Build history of the part. All positions in model axes, mm. Face numbers are marked on the shaded views. A direction names the side the tool comes from. Coordinates: 2 decimals unless noted, no trailing zeros. Loops run counter-clockwise (first coordinate to the right, second up) from the corner with the lowest first, then second, coordinate; pieces in that order, holes last. Notation, with made-up numbers: (39.5, -39) - (85.5, -39) arc R20 cw to (85.5, -4) - close; hole circle Ø3 at (-36, 86.25). An arc over 180 degrees is marked (long way). One line per item, written item: value.
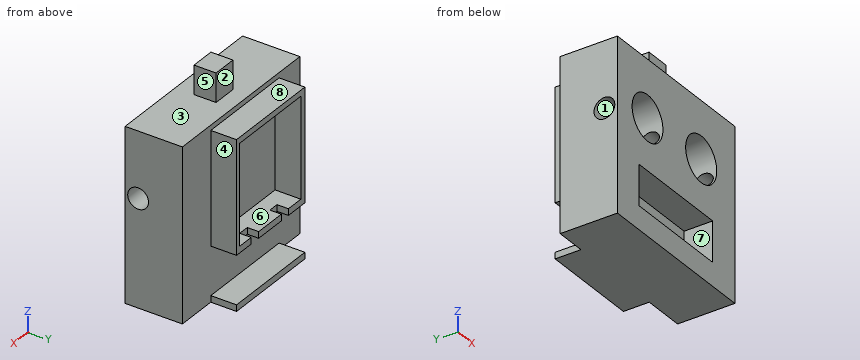
```python
from build123d import *

# Parameters (mm, degrees)
F0_W      = 76.2
F0_H      = 76.2
F1_DEPTH  = 25.4
F2_R      = 9.9906314399
F2_R_2    = 10.0773114698
F3_DEPTH  = 12.7
F4_W      = 47.7757537737
F4_H      = 17.8439570591
F5_DEPTH  = 12.7
F6_R      = 4.6109216101
F7_DEPTH  = 127
F8_W      = 44.3220883608
F8_H      = 49.7903954238
F9_DEPTH  = 11.43
F10_W     = 39.717190899
F10_H     = 44.3220883608
F11_DEPTH = 11.43
F12_W     = 44.3220883608
F12_H     = 2.8436683783
F13_DEPTH = 11.43
F14_W     = 4.6048909426
F14_H     = 2.8780568391
F14_W_2   = 4.8926984891
F15_DEPTH = 5.08
F16_W     = 10.9366197139
F16_H     = 9.7684562206
F17_DEPTH = 12.7


with BuildPart() as f1:
    # F0 (on Front) → F1 (new body)
    with BuildSketch(Plane.XZ):
        with Locations((-10.2171050385, 1.5830600848)):
            Rectangle(F0_W, F0_H)
    extrude(amount=-F1_DEPTH)

    # F2 (on face) → F3 (cut)
    with BuildSketch(Plane.XZ):
        with Locations((-28.7805758417, 14.3902888522)):
            Circle(F2_R)
        with Locations((6.0439212248, 14.3902888522)):
            Circle(F2_R_2)
    extrude(amount=-F3_DEPTH, mode=Mode.SUBTRACT)

    # F4 (on face) → F5 (cut)
    with BuildSketch(Plane.XZ):
        with Locations((-10.3610078804, -17.2683452256)):
            Rectangle(F4_W, F4_H)
    extrude(amount=-F5_DEPTH, mode=Mode.SUBTRACT)

    # F6 (on face) → F7 (cut)
    with BuildSketch(Plane.YZ.offset(27.8828949615)):
        with Locations((5.7532191277, 10.6449518353)):
            Circle(F6_R)
    extrude(amount=-F7_DEPTH, mode=Mode.SUBTRACT)

    # F8 (on face) → F9 (join)
    with BuildSketch(Plane(origin=(0, 25.4, 0), x_dir=(-1, 0, 0), z_dir=(0, 1, 0))):
        with Locations((12.6634538174, 12.5195505098)):
            Rectangle(F8_W, F8_H)
    extrude(amount=F9_DEPTH)

    # F10 (on face) → F11 (cut)
    with BuildSketch(Plane(origin=(0, 36.83, 0), x_dir=(-1, 0, 0), z_dir=(0, 1, 0))):
        with Locations((12.3756448738, 12.6634538174)):
            Rectangle(F10_W, F10_H)
    extrude(amount=-F11_DEPTH, mode=Mode.SUBTRACT)

    # F12 (on face) → F13 (join)
    with BuildSketch(Plane(origin=(0, 25.4, 0), x_dir=(-1, 0, 0), z_dir=(0, 1, 0))):
        with Locations((12.6634538174, -35.095105726)):
            Rectangle(F12_W, F12_H)
    extrude(amount=F13_DEPTH)

    # F14 (on face) → F15 (cut)
    with BuildSketch(Plane(origin=(0, 36.83, 0), x_dir=(-1, 0, 0), z_dir=(0, 1, 0))):
        with Locations((21.8732375652, -10.9366187826)):
            Rectangle(F14_W, F14_H)
        with Locations((2.4463492446, -10.9366187826)):
            Rectangle(F14_W_2, F14_H)
    extrude(amount=-F15_DEPTH, mode=Mode.SUBTRACT)

    # F16 (on face) → F17 (join)
    with BuildSketch(Plane.XY.offset(39.6830600848)):
        with Locations((-10.0732017308, 13.2293850183)):
            Rectangle(F16_W, F16_H)
    extrude(amount=F17_DEPTH)


solid = f1.part
```
Item 1: Probe probe 1 along X at (y, z) = (28.5, 32.5); probe 2 along X at (y, z) = (11, 22); probe 3 along Y at (x, z) = (-37, -14.5). List the from-to ranges inside material, lowest first. Write a range as from..to.
Check result:
probe 1: x = -34.82..-32.23, 7.48..9.5
probe 2: x = -48.32..-35.25, -22.31..-0.56, 12.65..27.88
probe 3: y = 0..25.4
Item 2: Tool access for the marked faces 4, 5, 6, 7 and 8: list every direction of +Z, -Z, +X, -X, +Y, -Y with a clear straight run to the whole face (end or side of a thin tool).
Check result:
face 4: +Z, -Z, +X, +Y
face 5: +Z, +X, +Y, -Y
face 6: +Y
face 7: -Y
face 8: +Z, +X, -X, +Y
Item 3: Cut at A-A, the plane y = 29. Write the cut outline in (x, z), then the cut area to 3 significant figures.
Check result:
outline: (-34.82, -36.52) - (9.5, -36.52) - (9.5, -33.67) - (-34.82, -33.67) - close; (-34.82, -12.38) - (9.5, -12.38) - (9.5, 37.41) - (-34.82, 37.41) - close; hole (-32.23, -9.5) - (7.48, -9.5) - (7.48, 34.82) - (-32.23, 34.82) - close
area: 573 mm^2
Item 4: Cut at D-D, the plane x = -6.5. Write the cut outline in (y, z), then the cut area to 3 significant figures.
Check result:
outline: (0, -36.52) - (36.83, -36.52) - (36.83, -33.67) - (25.4, -33.67) - (25.4, -12.38) - (36.83, -12.38) - (36.83, -9.5) - (25.4, -9.5) - (25.4, 34.82) - (36.83, 34.82) - (36.83, 37.41) - (25.4, 37.41) - (25.4, 39.68) - (18.11, 39.68) - (18.11, 52.38) - (8.35, 52.38) - (8.35, 39.68) - (0, 39.68) - (0, -8.35) - (12.7, -8.35) - (12.7, -26.19) - (0, -26.19) - close; hole circle Ø9.22 at (5.75, 10.64)
area: 1,860 mm^2
Item 5: Drop flat-ended pins along their axis: P1, Ø3.5, axis at x = -11.5, z = 45.5, coming from the +Y side; P2, Ø1.4, axis at y = 35, z = -10.5, coming from the -X side; P3, Ø2.5, axis at x = -3, z = -11.5, coming from the +Y side. Give the stop position or say it passes through.
Check result:
P1: stops at y = 18.11
P2: stops at x = -34.82
P3: stops at y = 31.75
Item 6: Cut at C-C, the plane z = -15. Write the cut outline in (x, y).
Check result:
outline: (-48.32, 0) - (-34.25, 0) - (-34.25, 12.7) - (13.53, 12.7) - (13.53, 0) - (27.88, 0) - (27.88, 25.4) - (-48.32, 25.4) - close
Item 7: Pull direction Y, two halves, no side cores. Call the marked faces 1, 2 and 3: released by +Y, released by -Y, zero draft, split by the parting line, or undercut.
Check result:
face 1: undercut
face 2: released by +Y
face 3: zero draft
Item 8: Cut at B-B, the plane y = 34.5. Write the cut outline in (x, z), then the cut area to 3 significant figures.
Check result:
outline: (-34.82, -36.52) - (9.5, -36.52) - (9.5, -33.67) - (-34.82, -33.67) - close; (-34.82, -12.38) - (-24.18, -12.38) - (-24.18, -9.5) - (-32.23, -9.5) - (-32.23, 34.82) - (7.48, 34.82) - (7.48, -9.5) - (0, -9.5) - (0, -12.38) - (9.5, -12.38) - (9.5, 37.41) - (-34.82, 37.41) - close; (-19.57, -12.38) - (-4.89, -12.38) - (-4.89, -9.5) - (-19.57, -9.5) - close
area: 545 mm^2
